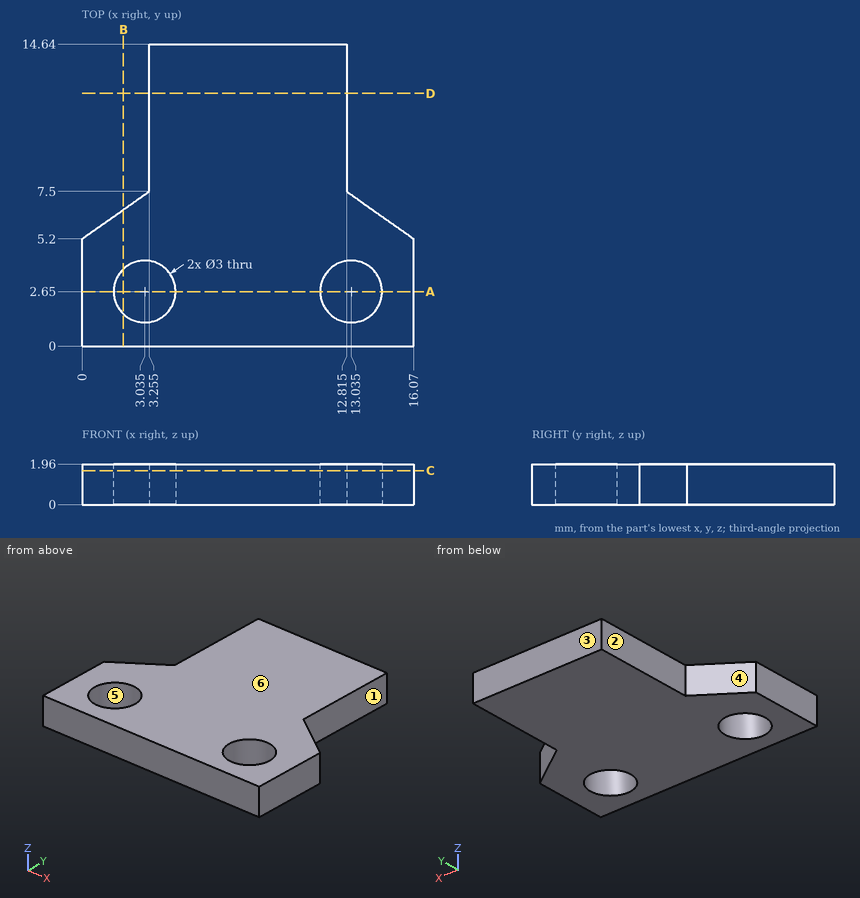
Part print with two shaded views. Sizes in mm from the minimum x, y, z corner. A direction names the side the tool comes from. Give positions to 0.01 mm unless a question says otherwise; leave off trailing zeros. Order: outer loops, then holes, each group sorted by start corner. A loop starts at its lowest first (then second) coordinate and runs counter-clockwise, first axis right, second up. Notation, with made-up numbers: M 54.25,18.25 L 74.25,18.25 A29 ccw 74.25,52.25 Z; hole C -40,41 d2. An arc over 180 degrees is marked long. Write item = value, one per line.
Q1. Cut at B-B, the plane x = 2. List the corners of the cut face in (y, z), then the cut area to 3 significant figures.
Derived:
outline = M 0,0 L 1.56,0 L 1.56,1.96 L 0,1.96 Z; M 3.74,0 L 6.61,0 L 6.61,1.96 L 3.74,1.96 Z
area = 8.71 mm2
Q2. Cut at C-C, the plane z = 1.65. List the corners of the cut face in (x, y) (3 decimals).
Derived:
outline = M 0,0 L 16.07,0 L 16.07,5.2 L 12.815,7.5 L 12.815,14.64 L 3.255,14.64 L 3.255,7.5 L 0,5.2 Z; hole C 3.035,2.65 d3; hole C 13.035,2.65 d3
Q3. Tool access for the marked faces 1, 2 and 3: list every direction of +Z, -Z, +X, -X, +Y, -Y with a clear straight run to the whole face (end or side of a thin tool).
Derived:
face_1 = +Z, -Z, +X, +Y
face_2 = +Z, -Z, -X, +Y
face_3 = +Z, -Z, +X, -X, +Y
Q4. Cut at A-A, the plane y = 2.65. List the corners of the cut face in (x, z) (3 decimals).
Derived:
outline = M 0,0 L 1.535,0 L 1.535,1.96 L 0,1.96 Z; M 4.535,0 L 11.535,0 L 11.535,1.96 L 4.535,1.96 Z; M 14.535,0 L 16.07,0 L 16.07,1.96 L 14.535,1.96 Z
Q5. Two-plate mould, pull along Y, no slides. Class the marked faces 4, 5 and 6: pulls with the +Y half, pulls with the -Y half, needs draft (parallel to the pull), parting line crosses it, or undercut.
Derived:
face_4 = pulls with the +Y half
face_5 = undercut
face_6 = needs draft
Q6. Cut at D-D, the plane y = 12.25. List the corners of the cut face in (x, z) (3 decimals).
Derived:
outline = M 3.255,0 L 12.815,0 L 12.815,1.96 L 3.255,1.96 Z
Q7. Flat gauge pins, fed straight in: pin 1 (0.6 mm diameter, centred on y = 9.5, z = 0.5, fed in from -X) (3 decimals); pin 2 (1 mm diameter, centred on y = 9, z = 1, fed in from +X) (3 decimals). Where does each tip first touch, or does it go through?
Derived:
pin_1 = 3.255
pin_2 = 12.815
Q8. Drill centre lines: line 1 (X direction, y = 2.75, z = 0.55); line 2 (X direction, y = 1.75, z = 0.5) (3 decimals); line 3 (X direction, y = 13.5, z = 0.9) (3 decimals). Where is each one in solid material? Low to high. Write a range as [from, to].
Derived:
line_1 = [0, 1.54], [4.53, 11.54], [14.53, 16.07]
line_2 = [0, 1.835], [4.235, 11.835], [14.235, 16.07]
line_3 = [3.255, 12.815]
